Autodesk Inventor part; units mm, degrees
ref_plane "YZ Plane" through (0, 0, 0) normal (1, 0, 0) x (0, 1, 0)
ref_plane "XZ Plane" through (0, 0, 0) normal (0, 1, 0) x (-1, 0, 0)
ref_plane "XY Plane" through (0, 0, 0) normal (0, 0, 1) x (1, 0, 0)
sketch "Sketch1" plane through (0, 0, 0) normal (0, 1, 0) x (-1, 0, 0)
  line L0 (99.05, 4.5) -> (-99.05, 4.5)
  line L1 (-99.05, 4.5) -> (-99.05, -4.5)
  line L2 (-99.05, -4.5) -> (99.05, -4.5)
  line L3 (99.05, -4.5) -> (99.05, 4.5)
  line L4 (99.05, 4.5) -> (-99.05, -4.5) construction
  line L5 (-99.05, 4.5) -> (99.05, -4.5) construction
  line L6 (99.05, 0) -> (87.55, 0) construction
  line L7 (-99.05, 0) -> (-87.55, 0) construction
  circle A0 centre (-87.55, 0) radius 1.5
  circle A1 centre (87.55, 0) radius 1.5
  line L8 (87.55, -1.5) -> (-87.55, -1.5)
  line L9 (99.05, 4.5) -> (99.05, 12.375)
  line L10 (99.05, 4.5) -> (106.925, 4.5) construction
  line L11 (99.05, 12.375) -> (94.05, 12.375)
  line L12 (94.05, 12.375) -> (94.05, 20.375)
  line L13 (94.05, 20.375) -> (99.05, 20.375)
  line L14 (99.05, 20.375) -> (99.05, 12.375)
  line L15 (94.05, 12.375) -> (94.05, 4.5)
  line L16 (94.05, 12.375) -> (101.925, 12.375) construction
  line L17 (-99.05, 4.5) -> (-99.05, 12.375)
  line L18 (-99.05, 4.5) -> (-91.175, 4.5) construction
  line L19 (-99.05, 12.375) -> (-94.05, 12.375)
  line L20 (-94.05, 12.375) -> (-94.05, 20.375)
  line L21 (-94.05, 20.375) -> (-99.05, 20.375)
  line L22 (-99.05, 20.375) -> (-99.05, 12.375)
  line L23 (-94.05, 12.375) -> (-94.05, 4.5)
  line L24 (-94.05, 12.375) -> (-86.175, 12.375) construction
  circle A2 centre (0, 0) radius 1.5
  line L25 (0, -1.5) -> (-8, -1.5) construction
  line L26 (0, -1.5) -> (8, -1.5) construction
  circle A3 centre (8, 0) radius 1.5
  circle A4 centre (-8, 0) radius 1.5
  line L27 (96.55, 20.375) -> (96.55, 17.375) construction
  line L28 (-96.55, 20.375) -> (-96.55, 17.375) construction
  circle A5 centre (-96.55, 17.375) radius 1.5
  circle A6 centre (96.55, 17.375) radius 1.5
  line L29 (87.55, 1.5) -> (-87.55, 1.5)
  point P0 (-94.05, 4.5)
  point P1 (8, -1.5)
  point P2 (-8, -1.5)
  point P3 (8.3564, -1.4534)
  point P4 (-7.6436, -1.4608)
  point P5 (-8, 1.5)
  point P6 (8, 1.5)
  dimension "d27" = 3
  dimension "d0" = 198.1
  dimension "d1" = 9
  dimension "d2" = 11.5
  dimension "d3" = 11.5
  dimension "d4" = 3
  dimension "d5" = 3
  dimension "d8" = 7.875
  dimension "d9" = 90
  dimension "d10" = 5
  dimension "d11" = 8
  dimension "d12" = 90
  dimension "d13" = 7.875
  dimension "d14" = 90
  dimension "d15" = 5
  dimension "d16" = 8
  dimension "d17" = 90
  dimension "d28" = 8
  dimension "d29" = 8
  dimension "d30" = 3
  dimension "d31" = 3
  dimension "d32" = 1.5
  dimension "d33" = 8
  dimension "d34" = 8
  dimension "d35" = 1.5
  dimension "d36" = 3
  dimension "d37" = 3
  dimension "d38" = 3
  dimension "d39" = 3
extrude "Extrusion1" add sketch "Sketch1" along normal blind 5 contours L3 L2 L1 L0 | L29 A2 L8 A4 | L29 A3 L8 A2 | A2
sketch "Sketch4" plane through (0, 5, 0) normal (0, 1, 0) x (1, 0, 0)
  line L0 (99.05, -4.5) -> (99.05, 4.5) construction
  line L1 (99.05, 0) -> (109.05, 0) construction
  line L2 (99.05, 0) -> (96.05, 0) construction
  line L3 (99.05, -1.5) -> (93.05, -1.5)
  line L4 (93.05, -1.5) -> (93.05, 1.5)
  line L5 (93.05, 1.5) -> (99.05, 1.5)
  line L6 (99.05, 1.5) -> (99.05, -1.5)
  line L7 (99.05, -1.5) -> (93.05, 1.5) construction
  line L8 (93.05, -1.5) -> (99.05, 1.5) construction
  line L9 (-99.05, 4.5) -> (-99.05, -4.5) construction
  line L10 (-99.05, 0) -> (-93.05, 0) construction
  line L11 (-99.05, -1.5) -> (-93.05, -1.5)
  line L12 (-93.05, -1.5) -> (-93.05, 1.5)
  line L13 (-93.05, 1.5) -> (-99.05, 1.5)
  line L14 (-99.05, 1.5) -> (-99.05, -1.5)
  line L15 (-99.05, -1.5) -> (-93.05, 1.5) construction
  line L16 (-93.05, -1.5) -> (-99.05, 1.5) construction
  point P0 (0, 0)
  point P1 (-96.05, 0)
  dimension "d54" = 3
  dimension "d55" = 6
  dimension "d56" = 3
  dimension "d57" = 6
  dimension "d58" = 6
  dimension "d59" = 3
extrude "Extrusion4" add sketch "Sketch4" along normal blind 14
sketch "Sketch5" plane through (-99.05, 5, 1.5) normal (0, 0, 1) x (1, 0, 0)
  line L0 (6, 14) -> (0, 14) construction
  line L1 (3, 14) -> (3, 11) construction
  circle A0 centre (3, 11) radius 1.5
  line L2 (198.1, 14) -> (192.1, 14) construction
  line L3 (195.1, 14) -> (195.1, 11) construction
  line L4 (195.1, 14) -> (198.1, 14) construction
  circle A1 centre (195.1, 11) radius 1.5
  point P0 (99.05, -5)
  dimension "d62" = 3
  dimension "d63" = 3
  dimension "d64" = 3
  dimension "d65" = 90
  dimension "d66" = 3
extrude "Extrusion5" cut sketch "Sketch5" against normal through all
fillet "Fillet4" radius 2 4 edges at (99.05, 19, 0) (93.05, 19, 0) (-93.05, 19, 0) (-99.05, 19, 0)
fillet "Fillet5" radius 2 10 edges at (-96.05, 5, 1.5) (-96.05, 5, -1.5) (-93.05, 5, 0) (96.05, 5, 1.5) (93.05, 5, 0) (96.05, 5, -1.5) (99.05, 2.5, 4.5) (99.05, 2.5, -4.5) (-99.05, 2.5, 4.5) (-99.05, 2.5, -4.5)
properties part number "Brace_slide_v3"
The model under review builds one solid part; all positions refer to its coordinate system, in mm. A direction names the side the tool comes from. Round coordinates to 2 decimals unless told otherwise and drop trailing zeros. Write each loop counter-clockwise with the first axis right and the second up, starting at its lowest first coordinate (ties: lowest second). Pieces come first, ordered by that corner, then holes.
(1) Mouldability with a two-part tool opening along X and no side actions: class faces 1 (the cylindrical face through (-89.05, 2.46, 0.03)), 2 (the flat face through (99.05, 6, 0)), 3 (the flat face through (96, 13, 1.5)) as +X half, -X half, draft (parallel to the pull), parting line (faces both ways), or undercut.
(2) Wall thickness on L1, parallel to Y at x = -96.05, z = -0.55; L2, parallel to X at y = 15, z = -0.5; L3, parallel to Z at x = 85.5, y = 2: over which ranges is each line inside the solid? List them lowest first.
(3) We need section B-B on x = -78. Give the boundary of the cut face in (y, z).
(4) We need section A-A on z = 0. Give the boundary of the cut face in (x, y).
(5) Insertion check: pin 1 (1.8 mm diameter, centred on x = -96.5, y = 13, fed in from -Z); pin 2 (4 mm diameter, centred on x = -12.5, z = -3, fed in from -Y); pin 3 (1.8 mm diameter, centred on x = 95, y = 10.5, fed in from +Z); pin 4 (2.5 mm diameter, centred on x = -4, z = -1.5, fed in from +Y). Each pin has a flat end and moves straight along its axis. Give the tip position at first contact, or say it passes through.
(6) Machinability: for faces 4 (the flat face through (96, 13, -1.5)), 5 (the flat face through (47, 2, -1.5)), 6 (the flat face through (-93.05, 12, 0)), 7 (the flat face through (-96, 13, 1.5)), 8 (the flat face through (1, 0, 0)), which of the approach directions +Z, -Z, +X, -X, +Y, -Y give a long, thin tool a straight path to every point of the face, cutting with its end or side? Answer none if there is none.
Findings below:
1. face 1: undercut
1. face 2: +X half
1. face 3: draft
2. L1: y = 0 to 14.5, 17.5 to 19
2. L2: x = -99.05 to -97.17, -94.93 to -93.05, 93.05 to 94.93, 97.17 to 99.05
2. L3: z = -4.5 to -1.5, 1.5 to 4.5
3. outline: (0, -4.5) - (5, -4.5) - (5, -1.5) - (0, -1.5) - close; (0, 1.5) - (5, 1.5) - (5, 4.5) - (0, 4.5) - close
4. outline: (-99.05, 0) - (-89.05, 0) - (-89.05, 5) - (-91.05, 5) arc R2 cw to (-93.05, 7) - (-93.05, 17) arc R2 ccw to (-95.05, 19) - (-97.05, 19) arc R2 ccw to (-99.05, 17) - close; (-6.5, 0) - (6.5, 0) - (6.5, 5) - (-6.5, 5) - close; (89.05, 0) - (99.05, 0) - (99.05, 17) arc R2 ccw to (97.05, 19) - (95.05, 19) arc R2 ccw to (93.05, 17) - (93.05, 7) arc R2 cw to (91.05, 5) - (89.05, 5) - close; hole circle Ø3 at (-96.05, 16); hole circle Ø3 at (96.05, 16)
5. pin 1: stops at z = -1.5
5. pin 2: stops at y = 0
5. pin 3: stops at z = 1.5
5. pin 4: stops at y = 5
6. face 4: -Z, +X, -X, +Y
6. face 5: +Y, -Y
6. face 6: +Z, -Z, +Y
6. face 7: +Z, +X, -X, +Y
6. face 8: +Z, -Z, +X, -X, -Y
